```python
from build123d import *

# Parameters (mm, degrees)
F0_W     = 82.55
F0_H     = 82.55
F0_W_2   = 31.75
F0_H_2   = 31.75
F1_DEPTH = 304.8
F2_R     = 38.1
F3_DEPTH = 304.8
F4_R     = 34.925
F4_R_2   = 30.48
F5_DEPTH = 762
F6_R     = 38.1
F6_R_2   = 30.48
F7_DEPTH = 3.175


with BuildPart() as f1:
    # F0 (on Front) → F1 (new body)
    with BuildSketch(Plane.XZ):
        with Locations((15.875, 15.875)):
            Rectangle(F0_W, F0_H)
        with Locations((15.875, 15.875)):
            Rectangle(F0_W_2, F0_H_2, mode=Mode.SUBTRACT)
    extrude(amount=-F1_DEPTH)

    # F2 (on face) → F3 (join)
    with BuildSketch(Plane(origin=(0, 304.8, 0), x_dir=(-1, 0, 0), z_dir=(0, 1, 0))):
        with BuildLine():
            ThreePointArc((-15.8749998581, -25.4), (13.3108324437, -13.3108323433), (25.4, 15.875))
            ThreePointArc((25.4, 15.875), (13.3108323935, 45.0608323935), (-15.875, 57.15))
            ThreePointArc((-15.875, 57.15), (-45.0608324126, 45.0608323743), (-57.15, 15.8749999458))
            ThreePointArc((-57.15, 15.8749999458), (-45.0608323241, -13.3108324628), (-15.8749998581, -25.4))
        make_face()
        with Locations((-15.875, 15.875)):
            Circle(F2_R, mode=Mode.SUBTRACT)
    extrude(amount=F3_DEPTH)



with BuildPart() as f5:
    # F4 (on face) → F5 (new body)
    with BuildSketch(Plane(origin=(0, 609.6, 0), x_dir=(-1, 0, 0), z_dir=(0, 1, 0))):
        with Locations((-15.875, 15.875)):
            Circle(F4_R)
        with Locations((-15.875, 15.875)):
            Circle(F4_R_2, mode=Mode.SUBTRACT)
    extrude(amount=F5_DEPTH)


with BuildPart() as f1_1:
    add(f1.part)

    add(f5.part)  # F7 merges F5
    # F6 (on face) → F7 (join, symmetric)
    with BuildSketch(Plane(origin=(0, 609.6, 0), x_dir=(-1, 0, 0), z_dir=(0, 1, 0))):
        with Locations((-15.875, 15.875)):
            Circle(F6_R)
        with Locations((-15.875, 15.875)):
            Circle(F6_R_2, mode=Mode.SUBTRACT)
    extrude(amount=F7_DEPTH, both=True)


solid = f1_1.part
```
Design review of the part built by this model. Coordinates are the model's own, in mm. A direction names the side the tool comes from. Coordinates: 2 decimals unless noted, no trailing zeros. Write each loop counter-clockwise with the first axis right and the second up, starting at its lowest first coordinate (ties: lowest second). Pieces come first, ordered by that corner, then holes.
1) Add section B-B (y = 929.5). Write out the cut boundary in (x, z) (3 decimals).
2) Mouldability with a two-part tool opening along X and no side actions: class faces 1 (the cylindrical face through (40.063, 983.656, -2.672)), 2 (the flat face through (47, 304.8, 49)), 3 (the flat face through (-25.4, 150, 15)) as +X half, -X half, draft (parallel to the pull), parting line (faces both ways), or undercut.
3) Insertion check: pin 1 (6 mm diameter, centred on x = 31, y = 318.5, fed in from +Z); pin 2 (8 mm diameter, centred on y = 1029.5, z = -3, fed in from -X); pin 3 (6 mm diameter, centred on x = 0.5, y = 600, fed in from -Z). Each pin has a flat end and moves straight along its axis. Give the tip position at first contact, or say it passes through.
4) Machinability: for faces 4 (the flat face through (33, 606.425, 41.5)), 5 (the cylindrical face through (43.59, 986.876, -5.376)), 6 (the flat face through (31.75, 150, 16)), which of the approach directions +Z, -Z, +X, -X, +Y, -Y give a long, thin tool a straight path to every point of the face, cutting with its end or side? Answer none if there is none.
5) To check wall thickness, follow L1, parallel to Y at x = 48, z = 8.5 (3 decimals); L2, parallel to X at y = 1285, z = 18; L3, parallel to X at y = 551, z = 15. State the ranges of each line that lie inside material, in increasing order.
6) Add section A-A (y = 279). Write out the cut boundary in (x, z).
Check result:
1. outline: circle Ø69.85 at (15.875, 15.875); hole circle Ø60.96 at (15.875, 15.875)
2. face 1: undercut
2. face 2: draft
2. face 3: -X half
3. pin 1: stops at z = 55.33
3. pin 2: stops at x = -15.72
3. pin 3: stops at z = -23.5
4. face 4: none
4. face 5: +Y
4. face 6: +Y, -Y
5. L1: y = 0 to 304.8, 606.425 to 1371.6
5. L2: x = -18.99 to -14.53, 46.28 to 50.74
5. L3: x = -25.39 to -22.21, 53.96 to 57.14
6. outline: (-25.4, -25.4) - (57.15, -25.4) - (57.15, 57.15) - (-25.4, 57.15) - close; hole (0, 0) - (31.75, 0) - (31.75, 31.75) - (0, 31.75) - close
